Part model, mm, in its own coordinate system. Round coordinates to 2 decimals unless told otherwise and drop trailing zeros. Loops run counter-clockwise (first coordinate to the right, second up) from the corner with the lowest first, then second, coordinate; pieces in that order, holes last. Notation, with made-up numbers: M 39,32 L 57,32 A29 cw 57,59 Z; hole C 7.5,34.5 d2. An arc over 180 degrees is marked long. Answer as CSV lines item,"result". Start each with the question number.
Item 1: Band-saw the part on C-C (y = -2.4). Give the cut face in (x, z), and give its area (3 significant figures).
Item 2: Band-saw the part on D-D (z = -17). Give the cut face in (x, y) (3 decimals), and give its area (3 significant figures).
Item 3: Wall check: line 1 (X direction, y = -2.5, z = 5.5); line 2 (Z direction, x = 1, y = -1.25); line 3 (Z direction, x = 15, y = -0.6). Give the ranges that are in metal, low to high.
Item 4: Band-saw the part on B-B (x = -16.5). Give the cut face in (y, z) (3 decimals).
Item 5: Band-saw the part on A-A (z = -2). Give the cut face in (x, y) (3 decimals).
```python
from build123d import *

# Parameters (mm, degrees)
F0_W     = 41.2496
F0_H     = 41.2496
F0_R     = 2.1463
F0_W_2   = 10.16
F0_H_2   = 22.86
F1_DEPTH = 3.175
F2_R     = 3.048
F3_R     = 0.5969


with BuildPart() as f1:
    # F0 (on Front) → F1 (new body)
    with BuildSketch(Plane.XZ):
        Rectangle(F0_W, F0_H)
        with Locations((-16.256, -15.494)):
            Circle(F0_R, mode=Mode.SUBTRACT)
        with Locations((16.256, -15.494)):
            Circle(F0_R, mode=Mode.SUBTRACT)
        with Locations((-16.256, 15.494)):
            Circle(F0_R, mode=Mode.SUBTRACT)
        Rectangle(F0_W_2, F0_H_2, mode=Mode.SUBTRACT)
        with Locations((16.256, 15.494)):
            Circle(F0_R, mode=Mode.SUBTRACT)
    extrude(amount=F1_DEPTH)

    # F2
    f2_edges = [f1.edges().sort_by_distance(p)[0] for p in [
        (20.6248, -1.5875, 20.6248),
        (-20.6248, -1.5875, 20.6248),
        (-20.6248, -1.5875, -20.6248),
        (20.6248, -1.5875, -20.6248),
    ]]
    fillet(f2_edges, radius=F2_R)

    # F3
    f3_edges = [f1.edges().sort_by_distance(p)[0] for p in [
        (-5.08, -1.5875, 11.43),
        (5.08, -1.5875, 11.43),
        (-5.08, -1.5875, -11.43),
        (5.08, -1.5875, -11.43),
    ]]
    fillet(f3_edges, radius=F3_R)


solid = f1.part
```
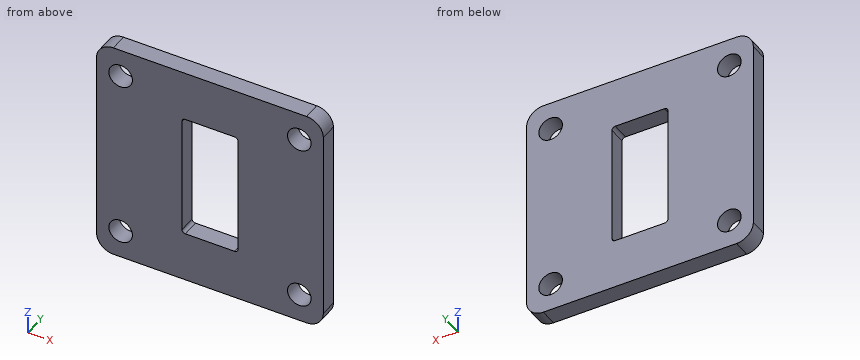
Answer block:
1,outline,"M -20.62,-17.58 A3.05 ccw -17.58,-20.62 L 17.58,-20.62 A3.05 ccw 20.62,-17.58 L 20.62,17.58 A3.05 ccw 17.58,20.62 L -17.58,20.62 A3.05 ccw -20.62,17.58 Z; hole C -16.26,-15.49 d4.29; hole C -16.26,15.49 d4.29; hole M -5.08,-10.83 A0.6 ccw -4.48,-11.43 L 4.48,-11.43 A0.6 ccw 5.08,-10.83 L 5.08,10.83 A0.6 ccw 4.48,11.43 L -4.48,11.43 A0.6 ccw -5.08,10.83 Z; hole C 16.26,-15.49 d4.29; hole C 16.26,15.49 d4.29"
1,area,"1,400 mm^2"
2,outline,"M -20.625,-3.175 L -17.785,-3.175 L -17.785,0 L -20.625,0 Z; M -14.727,-3.175 L 14.727,-3.175 L 14.727,0 L -14.727,0 Z; M 17.785,-3.175 L 20.625,-3.175 L 20.625,0 L 17.785,0 Z"
2,area,"112 mm^2"
3,line 1,"x = -20.62 to -5.08, 5.08 to 20.62"
3,line 2,"z = -20.62 to -11.43, 11.43 to 20.62"
3,line 3,"z = -20.62 to -17.23, -13.75 to 13.75, 17.23 to 20.62"
4,outline,"M -3.175,-20.625 L 0,-20.625 L 0,-17.626 L -3.175,-17.626 Z; M -3.175,-13.362 L 0,-13.362 L 0,13.362 L -3.175,13.362 Z; M -3.175,17.626 L 0,17.626 L 0,20.625 L -3.175,20.625 Z"
5,outline,"M -20.625,-3.175 L -5.08,-3.175 L -5.08,0 L -20.625,0 Z; M 5.08,-3.175 L 20.625,-3.175 L 20.625,0 L 5.08,0 Z"
